Here's how the part is built. I have some questions about the finished solid (model axes, mm). A direction names the side the tool comes from. Round coordinates to 2 decimals unless told otherwise and drop trailing zeros. Loops run counter-clockwise (first coordinate to the right, second up) from the corner with the lowest first, then second, coordinate; pieces in that order, holes last. Notation, with made-up numbers: M 42,-8.75 L 92,-8.75 A25 cw 92,16.25 Z; hole C 41.5,23 d2. An arc over 180 degrees is marked long. Use a Markdown table: item, result.
from build123d import *

# Parameters (mm, degrees)
SKETCH1_W           = 838.2
SKETCH1_H           = 711.2
BOSS_EXTRUDE1_DEPTH = 1397
SHELL1_T            = -2.54
CUT_EXTRUDE1_REACH  = 4.54
SKETCH2_W           = 833.12
SKETCH2_H           = 706.12


with BuildPart() as part:
    # Sketch1 → Boss-Extrude1 (new body)
    with BuildSketch(Plane(origin=(0, 0, 0), x_dir=(1, 0, 0), z_dir=(0, 1, 0))):
        with Locations((419.1, 355.6)):
            Rectangle(SKETCH1_W, SKETCH1_H)
    extrude(amount=BOSS_EXTRUDE1_DEPTH)

    # Shell1
    shell1_openings = [part.faces().sort_by_distance(p)[0] for p in [
        (419.1, 0, -355.6),
    ]]
    offset(amount=SHELL1_T, openings=shell1_openings, kind=Kind.INTERSECTION)

    # Sketch2 → Cut-Extrude1 (cut, up to next)
    with BuildSketch(Plane.XZ.offset(-1394.46), mode=Mode.PRIVATE) as cut_extrude1_sk1:
        with Locations((419.1, -355.6)):
            Rectangle(SKETCH2_W, SKETCH2_H)
    cut_extrude1_tool1 = extrude(cut_extrude1_sk1.sketch, amount=-CUT_EXTRUDE1_REACH, mode=Mode.PRIVATE) & part.part
    add(cut_extrude1_tool1.solids().sort_by_distance((419.1, 1394.46, -355.6))[0], mode=Mode.SUBTRACT)


solid = part.part
1. Which directions (+Z, -Z, +X, -X, +Y, -Y) give clear straight access to the entire face, cutting with the end or side of a thin tool? Please do faces 4 (the face through (413, 689, -711.2)), 5 (the face through (413, 689, -2.54)).
Answer sheet:
| item | result |
|---|---|
| face 4 | -Z, +X, -X, +Y, -Y |
| face 5 | +Y, -Y |
2. I need wall thicknesses on probe 1 along Z at (x, y) = (353, 122); probe 2 along X at (y, z) = (946.5, -446). Which ranges of each line are inside material? Lowest first, please. Write a range as from..to.
Answer sheet:
| item | result |
|---|---|
| probe 1 | -711.2..-708.66, -2.54..0 |
| probe 2 | 0..2.54, 835.66..838.2 |
3. We'd pull the mould along X, two halves only. Please class faces 1 (the face through (838.2, 689, -351)), 2 (the face through (413, 689, 0)), 3 (the face through (2.54, 689, -351)): +X half, -X half, draft (parallel to the pull), parting line (faces both ways), or undercut.
Answer sheet:
| item | result |
|---|---|
| face 1 | +X half |
| face 2 | draft |
| face 3 | undercut |
4. Imagine slicing it at A-A, the plane x = 135. Write out the boundary of the cut face in (y, z).
Answer sheet:
| item | result |
|---|---|
| outline | M 0,-711.2 L 1397,-711.2 L 1397,-708.66 L 0,-708.66 Z; M 0,-2.54 L 1397,-2.54 L 1397,0 L 0,0 Z |
5. Imagine slicing it at B-B, the plane y = 1297.5. Write out the boundary of the cut face in (x, z), then the cut area to 3 significant figures.
Answer sheet:
| item | result |
|---|---|
| outline | M 0,-711.2 L 838.2,-711.2 L 838.2,0 L 0,0 Z; hole M 2.54,-708.66 L 835.66,-708.66 L 835.66,-2.54 L 2.54,-2.54 Z |
| area | 7,850 mm2 |
6. Imagine slicing it at C-C, the plane z = -288. Write out the boundary of the cut face in (x, y), then the cut area to 3 significant figures.
Answer sheet:
| item | result |
|---|---|
| outline | M 0,0 L 2.54,0 L 2.54,1397 L 0,1397 Z; M 835.66,0 L 838.2,0 L 838.2,1397 L 835.66,1397 Z |
| area | 7,100 mm2 |
